Autodesk Inventor part; units mm, degrees
ref_plane "YZ Plane" through (0, 0, 0) normal (1, 0, 0) x (0, 1, 0)
ref_plane "XZ Plane" through (0, 0, 0) normal (0, 1, 0) x (-1, 0, 0)
ref_plane "XY Plane" through (0, 0, 0) normal (0, 0, 1) x (1, 0, 0)
sketch "Sketch1" plane through (0, 0, 0) normal (1, 0, 0) x (0, 1, 0)
  line L0 (-3.4784, 6.7709) -> (-9.8284, 6.7709)
  line L1 (-9.8284, 6.7709) -> (-9.8284, -5.9291)
  line L2 (-9.8284, -5.9291) -> (-3.4784, -5.9291)
  line L3 (-3.4784, -5.9291) -> (-3.4784, 6.7709)
  line L4 (-9.8092, -5.9291) -> (2.8908, -5.9291)
  line L5 (2.8908, -5.9291) -> (2.8908, 0.4209)
  line L6 (2.8908, 0.4209) -> (-9.8092, 0.4209)
  line L7 (-9.8092, 0.4209) -> (-9.8092, -5.9291)
  line L8 (2.8908, 0.4209) -> (21.9408, 0.4209)
  line L9 (21.9408, 0.4209) -> (21.9408, -5.9291)
  line L10 (21.9408, -5.9291) -> (2.8908, -5.9291)
  line L11 (2.8908, -5.9291) -> (2.8908, 0.4209)
  line L12 (21.9408, 0.4209) -> (9.2408, 0.4209)
  line L13 (9.2408, 0.4209) -> (9.2408, -18.6291)
  line L14 (9.2408, -18.6291) -> (21.9408, -18.6291)
  line L15 (21.9408, -18.6291) -> (21.9408, 0.4209)
  point P0 (0, 0)
  dimension "d0" = 6.35
  dimension "d1" = 12.7
  dimension "d2" = 12.7
  dimension "d3" = 6.35
  dimension "d4" = 19.05
  dimension "d5" = 6.35
  dimension "d6" = 12.7
  dimension "d7" = 19.05
extrude "Extrusion1" add sketch "Sketch1" along normal blind 50.8 contours L3 L6 L7 L2 L1 L0 | L3 L2 L7 L6
extrude "Extrusion2" add sketch "Sketch1" along normal blind 31.75 contours L8 L13 L10 L5 | L8 L9 L10 L13
extrude "Extrusion3" cut sketch "Sketch1" along normal blind 50.8 contours L6 L5 L4 L3 | L3 L2 L7 L6
extrude "Extrusion4" add sketch "Sketch1" along normal blind 50.8 contours L6 L5 L4 L3 | L3 L2 L7 L6
extrude "Extrusion5" cut sketch "Sketch1" along normal blind 31.75 contours L8 L9 L10 L13 | L10 L15 L14 L13
extrude "Extrusion6" add sketch "Sketch1" along normal blind 31.75 contours L8 L9 L10 L13 | L10 L15 L14 L13
sketch "Sketch2" plane through (0, 21.9408, 0.4209) normal (0, 1, 0) x (1, 0, 0)
  line L0 (31.75, 12.7) -> (31.75, 19.05)
  circle A0 centre (25.4, 12.7) radius 3.175
  point P0 (0, 0.4209)
  dimension "d22" = 6.35
extrude "Extrusion7" cut sketch "Sketch2" against normal blind 12.7
sketch "Sketch3" plane through (0, -3.4784, 0.4209) normal (0, 0, 1) x (1, 0, 0)
  line L0 (0, 12.7192) -> (0, 25.4192)
  line L1 (0, 25.4192) -> (6.35, 25.4192)
  line L2 (0, 19.0692) -> (0, 25.4192)
  line L3 (6.35, 25.4192) -> (9.525, 25.4192)
  line L4 (9.525, 19.0692) -> (6.35, 19.0692)
  circle A0 centre (9.525, 19.0692) radius 3.175
  point P0 (0, 3.4784)
  dimension "d27" = 3.175
  dimension "d28" = 6.35
  dimension "d29" = 6.35
extrude "Extrusion8" cut sketch "Sketch3" against normal blind 25.4
Input: part model. Units: mm. Frame: model coordinates. A direction names the side the tool comes from. Round coordinates to 2 decimals unless told otherwise and drop trailing zeros. Order: outer loops, then holes, each group sorted by start corner. A loop starts at its lowest first (then second) coordinate and runs counter-clockwise, first axis right, second up. Notation, with made-up numbers: (-10.75, -26) - (43.25, -26) arc R22 cw to (43.25, -5) - close; hole circle Ø7 at (8.5, -32). An arc over 180 degrees is marked (long way). Use a Markdown table: item, result.
1. Section D-D on y = 11. Return the cut outline in (x, z) (3 decimals), then the cut area to 3 significant figures.
Evaluation:
| item | result |
|---|---|
| outline | (0, -18.629) - (31.75, -18.629) - (31.75, 0.421) - (0, 0.421) - close; hole circle Ø6.35 at (25.4, -12.279) |
| area | 573 mm^2 |
2. Section A-A on x = 25.4. Return the cut outline in (y, z), then the cut area to 3 significant figures.
Evaluation:
| item | result |
|---|---|
| outline | (-9.83, -5.93) - (9.24, -5.93) - (9.24, -9.1) - (21.94, -9.1) - (21.94, 0.42) - (-3.48, 0.42) - (-3.48, 6.77) - (-9.83, 6.77) - close; (9.24, -18.63) - (21.94, -18.63) - (21.94, -15.45) - (9.24, -15.45) - close |
| area | 323 mm^2 |
3. Section C-C on x = 20. Return the cut outline in (y, z), then the cut area to 3 significant figures.
Evaluation:
| item | result |
|---|---|
| outline | (-9.83, -5.93) - (9.24, -5.93) - (9.24, -18.63) - (21.94, -18.63) - (21.94, 0.42) - (-3.48, 0.42) - (-3.48, 6.77) - (-9.83, 6.77) - close |
| area | 403 mm^2 |
4. First-contact query: pin 1 (7.5 mm diameter, centred on x = 34.5, y = 4.5, fed in from +Z); pin 2 (6 mm diameter, centred on x = 7.5, z = -10, fed in from -Y); pin 3 (15 mm diameter, centred on y = 16.5, z = -5.5, fed in from +X). Flat tips, straight axial feed; report the tip coordinate or a pass-through.
Evaluation:
| item | result |
|---|---|
| pin 1 | z = 0.42 |
| pin 2 | y = 9.24 |
| pin 3 | x = 31.75 |
5. Material intervals for probe 1 along Y at (x, z) = (34.5, 1.5); probe 2 along Z at (x, y) = (10.5, 4); probe 3 along Z at (x, y) = (34, -6), sorted ascending.
Evaluation:
| item | result |
|---|---|
| probe 1 | -9.83 to -3.48 |
| probe 2 | -5.93 to 0.42 |
| probe 3 | -5.93 to 6.77 |
6. Section B-B on z = -11.5. Return the cut outline in (x, y) (3 decimals), then the cut area to 3 significant figures.
Evaluation:
| item | result |
|---|---|
| outline | (0, 9.241) - (22.322, 9.241) - (22.322, 21.941) - (0, 21.941) - close; (28.478, 9.241) - (31.75, 9.241) - (31.75, 21.941) - (28.478, 21.941) - close; hole circle Ø6.35 at (9.525, 15.591) |
| area | 293 mm^2 |
7. Access query for faces 1 (the face through (25, -3.478, 4)), 2 (the face through (16, 9.241, -12)), 3 (the face through (50.8, -5, -1)), 4 (the face through (41, 2.891, -3)), 5 (the face through (25, -9.828, 1)). Directions: +Z, -Z, +X, -X, +Y, -Y. A direction counts if a zero-diameter tool reaches every point of the face in a straight line with its end or side. Return the directions, or none.
Evaluation:
| item | result |
|---|---|
| face 1 | +Z, +X, -X, +Y |
| face 2 | -Z, +X, -X, -Y |
| face 3 | +Z, -Z, +X, +Y, -Y |
| face 4 | +Z, -Z, +X, +Y |
| face 5 | +Z, -Z, +X, -X, -Y |
8. Mould query, pull axis X, two halves, no side actions, for faces 6 (the face through (28.43, 15.68, -13.23)), 7 (the face through (19, 9, 0.421)), 8 (the face through (31.75, 14, -9)). Classes: +X half, -X half, draft (parallel to the pull), parting line (faces both ways), or undercut.
Evaluation:
| item | result |
|---|---|
| face 6 | undercut |
| face 7 | draft |
| face 8 | +X half |
